The model under review builds one solid part; all positions refer to its coordinate system, in mm. A direction names the side the tool comes from. Coordinates: 2 decimals unless noted, no trailing zeros. Order: outer loops, then holes, each group sorted by start corner. A loop starts at its lowest first (then second) coordinate and runs counter-clockwise, first axis right, second up. Notation, with made-up numbers: (-19.5, 58.5) -> (20.5, 58.5) arc R16 ccw to (20.5, 77.5) -> close; hole circle Ø9 at (-0.75, 58.5). An arc over 180 degrees is marked (long way). Put each result on its own line as item: value.
from build123d import *

# Parameters (mm, degrees)
SKETCH1_W           = 310
SKETCH1_H           = 290
BOSS_EXTRUDE1_DEPTH = 10
CUT_EXTRUDE1_DEPTH  = 213.485293609
CUT_EXTRUDE2_DEPTH  = 186.337530006


with BuildPart() as part:
    # Sketch1 → Boss-Extrude1 (new body)
    with BuildSketch(Plane(origin=(0, 0, 0), x_dir=(1, 0, 0), z_dir=(0, 1, 0))):
        Rectangle(SKETCH1_W, SKETCH1_H)
    extrude(amount=BOSS_EXTRUDE1_DEPTH)

    # Sketch2 → Cut-Extrude1 (cut, through all)
    with BuildSketch(Plane(origin=(0, 10, 0), x_dir=(1, 0, 0), z_dir=(0, 1, 0))):
        Polygon((-85.000000124, 145), (-115.000000124, 87.499999968), (-115.000000124, -87.500000032), (-85, -145), (-155, -145), (-155.000000124, 144.999999996), align=None)
        Polygon((155, -145), (155.000000124, 144.999999996), (85.000000124, 145), (115.000000124, 87.499999968), (115.000000124, -87.500000032), (85, -145), align=None)
    extrude(amount=-CUT_EXTRUDE1_DEPTH, mode=Mode.SUBTRACT)

    # Sketch3 → Cut-Extrude2 (cut, through all)
    with BuildSketch(Plane.XZ):
        Polygon((-75.000000124, -145), (-75.000000124, -120), (-22.500000124, -120), (-22.500000124, 120), (-75.407979447, 120), (-75.407979447, 145), (-85, 145), (-115.000000124, 87.500000032), (-115.000000124, -87.499999968), (-85.000000124, -145), align=None)
        Polygon((75.000000124, -120), (22.500000124, -120), (22.500000124, 120), (75.407979447, 120), (75.407979447, 145), (85, 145), (115.000000124, 87.500000032), (115.000000124, -87.499999968), (85.000000124, -145), (75.000000124, -145), align=None)
    extrude(amount=-CUT_EXTRUDE2_DEPTH, mode=Mode.SUBTRACT)


solid = part.part
Item 1: Consider section B-B on y = 2.75. Write out the cut boundary in (x, z), and give its area (3 significant figures).
Answers below:
outline: (-75.41, 120) -> (-22.5, 120) -> (-22.5, -120) -> (-75, -120) -> (-75, -145) -> (75, -145) -> (75, -120) -> (22.5, -120) -> (22.5, 120) -> (75.41, 120) -> (75.41, 145) -> (-75.41, 145) -> close
area: 18,300 mm^2
Item 2: For faces 1 (the flat face through (-75, 5, -133)), 2 (the flat face through (49, 5, -120)), 3 (the flat face through (-1, 10, -2)), 4 (the flat face through (-49, 5, -120)), list the 3-axis set-ups (+Z, -Z, +X, -X, +Y, -Y) from which the entire face can be reached by the end or side of a thin tool; tool diameter is ignored.
Answers below:
face 1: -Z, -X, +Y, -Y
face 2: +X, +Y, -Y
face 3: +Z, -Z, +X, -X, +Y
face 4: -X, +Y, -Y
Item 3: For pin 1 Ø6 at (y, z) = (1, 97) entering from +X, flat-tipped, find the tip position at first contact; note if it passes through.
Answers below:
pin 1: x = 22.5
Item 4: Mouldability with a two-part tool opening along Z and no side actions: class faces 5 (the flat face through (-22.5, 5, -2)), 6 (the flat face through (-1, 5, 145)), 7 (the flat face through (75, 5, -133)) as +Z half, -Z half, draft (parallel to the pull), parting line (faces both ways), or undercut.
Answers below:
face 5: undercut
face 6: +Z half
face 7: draft
Item 5: Consider section C-C on z = -88.5. Write out the cut boundary in (x, y).
Answers below:
outline: (-22.5, 0) -> (22.5, 0) -> (22.5, 10) -> (-22.5, 10) -> close
Item 6: For line 1 (Z direction, x = -30.5, y = 7.5); line 2 (X direction, y = 1.25, z = 61), list the stretches that pass through material, from the lowest coordinate up. Write a range as from..to.
Answers below:
line 1: -145..-120, 120..145
line 2: -22.5..22.5
Item 7: Consider section A-A on x = 51.5. Write out the cut boundary in (y, z).
Answers below:
outline: (0, -145) -> (10, -145) -> (10, -120) -> (0, -120) -> close; (0, 120) -> (10, 120) -> (10, 145) -> (0, 145) -> close
